```python
from build123d import *

# Parameters (mm, degrees)
BOSS_EXTRU_1_DEPTH      = 80
CONG_1_R                = 3
CONG_2_R                = 5
ENL_V_MAT_EXTRU_1_REACH = 119.218
ESQUISSE2_R             = 2.75
ENL_V_MAT_EXTRU_2_REACH = 116.084
ESQUISSE3_R             = 6.25
ENL_V_MAT_EXTRU_3_REACH = 125.629
ESQUISSE4_R             = 2.75
ENL_V_MAT_EXTRU_4_REACH = 122.661
ESQUISSE5_R             = 6.25
ENL_V_START             = -3.408092413
ENL_V_MAT_EXTRU_5_DEPTH = 3.408092413


# Read off the part's stored shape, not the designer's step: Enlèv. mat.-Extru.5
with BuildPart() as part:
    # Esquisse1 → Boss.-Extru.1 (new body)
    with BuildSketch(Plane.XY):
        Polygon((-33.585720943, 17.910660079), (-33.585720943, -57.089339921), (-28.585720943, -57.089339921), (41.414279057, 12.910660079), (41.414279057, 17.910660079), align=None)
        Polygon((-28.585720943, -52.269569409), (-28.585720943, 12.910660079), (36.594508545, 12.910660079), align=None, mode=Mode.SUBTRACT)
    extrude(amount=BOSS_EXTRU_1_DEPTH)

    # Congé1
    cong_1_edges = [part.edges().sort_by_distance(p)[0] for p in [
        (-28.585720943, -52.269569409, 40),
        (36.594508545, 12.910660079, 40),
    ]]
    fillet(cong_1_edges, radius=CONG_1_R)

    # Congé2
    cong_2_edges = [part.edges().sort_by_distance(p)[0] for p in [
        (-28.585720943, 12.910660079, 40),
    ]]
    fillet(cong_2_edges, radius=CONG_2_R)

    # Esquisse2 → Enlèv. mat.-Extru.1 (cut, up to next)
    with BuildSketch(Plane(origin=(0, 17.910660079, 0), x_dir=(1, 0, 0), z_dir=(0, 1, 0)), mode=Mode.PRIVATE) as enl_v_mat_extru_1_sk1:
        with Locations(Location((-13.585720943, -10, 0), (0, 0, 180))):
            Circle(ESQUISSE2_R)
    enl_v_mat_extru_1_tool1 = extrude(enl_v_mat_extru_1_sk1.sketch, amount=-ENL_V_MAT_EXTRU_1_REACH, mode=Mode.PRIVATE) & part.part
    # Esquisse2 → Enlèv. mat.-Extru.1 (cut, up to next)
    with BuildSketch(Plane(origin=(0, 17.910660079, 0), x_dir=(1, 0, 0), z_dir=(0, 1, 0)), mode=Mode.PRIVATE) as enl_v_mat_extru_1_sk2:
        with Locations(Location((31.414279057, -10, 0), (0, 0, 180))):
            Circle(ESQUISSE2_R)
    enl_v_mat_extru_1_tool2 = extrude(enl_v_mat_extru_1_sk2.sketch, amount=-ENL_V_MAT_EXTRU_1_REACH, mode=Mode.PRIVATE) & part.part
    # Esquisse2 → Enlèv. mat.-Extru.1 (cut, up to next)
    with BuildSketch(Plane(origin=(0, 17.910660079, 0), x_dir=(1, 0, 0), z_dir=(0, 1, 0)), mode=Mode.PRIVATE) as enl_v_mat_extru_1_sk3:
        with Locations(Location((31.414279057, -70, 0), (0, 0, 180))):
            Circle(ESQUISSE2_R)
    enl_v_mat_extru_1_tool3 = extrude(enl_v_mat_extru_1_sk3.sketch, amount=-ENL_V_MAT_EXTRU_1_REACH, mode=Mode.PRIVATE) & part.part
    # Esquisse2 → Enlèv. mat.-Extru.1 (cut, up to next)
    with BuildSketch(Plane(origin=(0, 17.910660079, 0), x_dir=(1, 0, 0), z_dir=(0, 1, 0)), mode=Mode.PRIVATE) as enl_v_mat_extru_1_sk4:
        with Locations(Location((-13.585720943, -70, 0), (0, 0, 180))):
            Circle(ESQUISSE2_R)
    enl_v_mat_extru_1_tool4 = extrude(enl_v_mat_extru_1_sk4.sketch, amount=-ENL_V_MAT_EXTRU_1_REACH, mode=Mode.PRIVATE) & part.part
    add(enl_v_mat_extru_1_tool1.solids().sort_by_distance((-13.585721, 17.91066, 10))[0], mode=Mode.SUBTRACT)
    add(enl_v_mat_extru_1_tool2.solids().sort_by_distance((31.414279, 17.91066, 10))[0], mode=Mode.SUBTRACT)
    add(enl_v_mat_extru_1_tool3.solids().sort_by_distance((31.414279, 17.91066, 70))[0], mode=Mode.SUBTRACT)
    add(enl_v_mat_extru_1_tool4.solids().sort_by_distance((-13.585721, 17.91066, 70))[0], mode=Mode.SUBTRACT)

    # Enlèv. mat.-Extru.2: up to this plane
    enl_v_mat_extru_2_end = Plane(origin=(-28.585720943, -57.089339921, 80), z_dir=(-0.7071067811865477, 0.7071067811865474, 0))
    # Esquisse3 → Enlèv. mat.-Extru.2 (cut, up to the surface)
    with BuildSketch(Plane.XZ.offset(-12.910660079), mode=Mode.PRIVATE) as enl_v_mat_extru_2_sk1:
        with Locations((-13.585720943, 10)):
            Circle(ESQUISSE3_R)
    enl_v_mat_extru_2_tool1 = split(extrude(enl_v_mat_extru_2_sk1.sketch, amount=ENL_V_MAT_EXTRU_2_REACH, mode=Mode.PRIVATE), bisect_by=enl_v_mat_extru_2_end, keep=Keep.BOTH, mode=Mode.PRIVATE)
    add(enl_v_mat_extru_2_tool1.solids().sort_by_distance((-13.585721, 12.91066, 10))[0], mode=Mode.SUBTRACT)
    # Esquisse3 → Enlèv. mat.-Extru.2 (cut, up to the surface)
    with BuildSketch(Plane.XZ.offset(-12.910660079), mode=Mode.PRIVATE) as enl_v_mat_extru_2_sk2:
        with Locations((-13.585720943, 70)):
            Circle(ESQUISSE3_R)
    enl_v_mat_extru_2_tool2 = split(extrude(enl_v_mat_extru_2_sk2.sketch, amount=ENL_V_MAT_EXTRU_2_REACH, mode=Mode.PRIVATE), bisect_by=enl_v_mat_extru_2_end, keep=Keep.BOTH, mode=Mode.PRIVATE)
    add(enl_v_mat_extru_2_tool2.solids().sort_by_distance((-13.585721, 12.91066, 70))[0], mode=Mode.SUBTRACT)
    # Esquisse3 → Enlèv. mat.-Extru.2 (cut, up to the surface)
    with BuildSketch(Plane.XZ.offset(-12.910660079), mode=Mode.PRIVATE) as enl_v_mat_extru_2_sk3:
        with Locations(Location((31.414279057, 10, 0), (0, 0, 109.267913115))):
            Circle(ESQUISSE3_R)
    enl_v_mat_extru_2_tool3 = split(extrude(enl_v_mat_extru_2_sk3.sketch, amount=ENL_V_MAT_EXTRU_2_REACH, mode=Mode.PRIVATE), bisect_by=enl_v_mat_extru_2_end, keep=Keep.BOTH, mode=Mode.PRIVATE)
    add(enl_v_mat_extru_2_tool3.solids().sort_by_distance((31.414279, 12.91066, 10))[0], mode=Mode.SUBTRACT)
    # Esquisse3 → Enlèv. mat.-Extru.2 (cut, up to the surface)
    with BuildSketch(Plane.XZ.offset(-12.910660079), mode=Mode.PRIVATE) as enl_v_mat_extru_2_sk4:
        with Locations(Location((31.414279057, 70, 0), (0, 0, 109.267913115))):
            Circle(ESQUISSE3_R)
    enl_v_mat_extru_2_tool4 = split(extrude(enl_v_mat_extru_2_sk4.sketch, amount=ENL_V_MAT_EXTRU_2_REACH, mode=Mode.PRIVATE), bisect_by=enl_v_mat_extru_2_end, keep=Keep.BOTH, mode=Mode.PRIVATE)
    add(enl_v_mat_extru_2_tool4.solids().sort_by_distance((31.414279, 12.91066, 70))[0], mode=Mode.SUBTRACT)

    # Esquisse4 → Enlèv. mat.-Extru.3 (cut, up to next)
    with BuildSketch(Plane.ZY.offset(33.585720943), mode=Mode.PRIVATE) as enl_v_mat_extru_3_sk1:
        with Locations(Location((10, -47.089339921, 0), (0, 0, 270))):
            Circle(ESQUISSE4_R)
    enl_v_mat_extru_3_tool1 = extrude(enl_v_mat_extru_3_sk1.sketch, amount=-ENL_V_MAT_EXTRU_3_REACH, mode=Mode.PRIVATE) & part.part
    # Esquisse4 → Enlèv. mat.-Extru.3 (cut, up to next)
    with BuildSketch(Plane.ZY.offset(33.585720943), mode=Mode.PRIVATE) as enl_v_mat_extru_3_sk2:
        with Locations(Location((10, -2.089339921, 0), (0, 0, 270))):
            Circle(ESQUISSE4_R)
    enl_v_mat_extru_3_tool2 = extrude(enl_v_mat_extru_3_sk2.sketch, amount=-ENL_V_MAT_EXTRU_3_REACH, mode=Mode.PRIVATE) & part.part
    # Esquisse4 → Enlèv. mat.-Extru.3 (cut, up to next)
    with BuildSketch(Plane.ZY.offset(33.585720943), mode=Mode.PRIVATE) as enl_v_mat_extru_3_sk3:
        with Locations(Location((70, -2.089339921, 0), (0, 0, 270))):
            Circle(ESQUISSE4_R)
    enl_v_mat_extru_3_tool3 = extrude(enl_v_mat_extru_3_sk3.sketch, amount=-ENL_V_MAT_EXTRU_3_REACH, mode=Mode.PRIVATE) & part.part
    # Esquisse4 → Enlèv. mat.-Extru.3 (cut, up to next)
    with BuildSketch(Plane.ZY.offset(33.585720943), mode=Mode.PRIVATE) as enl_v_mat_extru_3_sk4:
        with Locations(Location((70, -47.089339921, 0), (0, 0, 270))):
            Circle(ESQUISSE4_R)
    enl_v_mat_extru_3_tool4 = extrude(enl_v_mat_extru_3_sk4.sketch, amount=-ENL_V_MAT_EXTRU_3_REACH, mode=Mode.PRIVATE) & part.part
    add(enl_v_mat_extru_3_tool1.solids().sort_by_distance((-33.585721, -47.08934, 10))[0], mode=Mode.SUBTRACT)
    add(enl_v_mat_extru_3_tool2.solids().sort_by_distance((-33.585721, -2.08934, 10))[0], mode=Mode.SUBTRACT)
    add(enl_v_mat_extru_3_tool3.solids().sort_by_distance((-33.585721, -2.08934, 70))[0], mode=Mode.SUBTRACT)
    add(enl_v_mat_extru_3_tool4.solids().sort_by_distance((-33.585721, -47.08934, 70))[0], mode=Mode.SUBTRACT)

    # Esquisse5 → Enlèv. mat.-Extru.4 (cut, up to next)
    with BuildSketch(Plane(origin=(-28.585720943, 0, 0), x_dir=(0, 0, -1), z_dir=(1, 0, 0)), mode=Mode.PRIVATE) as enl_v_mat_extru_4_sk1:
        with Locations((-10, -2.089339921)):
            Circle(ESQUISSE5_R)
    enl_v_mat_extru_4_tool1 = extrude(enl_v_mat_extru_4_sk1.sketch, amount=ENL_V_MAT_EXTRU_4_REACH, mode=Mode.PRIVATE) & part.part
    # Esquisse5 → Enlèv. mat.-Extru.4 (cut, up to next)
    with BuildSketch(Plane(origin=(-28.585720943, 0, 0), x_dir=(0, 0, -1), z_dir=(1, 0, 0)), mode=Mode.PRIVATE) as enl_v_mat_extru_4_sk2:
        with Locations((-70, -2.089339921)):
            Circle(ESQUISSE5_R)
    enl_v_mat_extru_4_tool2 = extrude(enl_v_mat_extru_4_sk2.sketch, amount=ENL_V_MAT_EXTRU_4_REACH, mode=Mode.PRIVATE) & part.part
    # Esquisse5 → Enlèv. mat.-Extru.4 (cut, up to next)
    with BuildSketch(Plane(origin=(-28.585720943, 0, 0), x_dir=(0, 0, -1), z_dir=(1, 0, 0)), mode=Mode.PRIVATE) as enl_v_mat_extru_4_sk3:
        with Locations((-10, -47.089339921)):
            Circle(ESQUISSE5_R)
    enl_v_mat_extru_4_tool3 = extrude(enl_v_mat_extru_4_sk3.sketch, amount=ENL_V_MAT_EXTRU_4_REACH, mode=Mode.PRIVATE) & part.part
    # Esquisse5 → Enlèv. mat.-Extru.4 (cut, up to next)
    with BuildSketch(Plane(origin=(-28.585720943, 0, 0), x_dir=(0, 0, -1), z_dir=(1, 0, 0)), mode=Mode.PRIVATE) as enl_v_mat_extru_4_sk4:
        with Locations((-70, -47.089339921)):
            Circle(ESQUISSE5_R)
    enl_v_mat_extru_4_tool4 = extrude(enl_v_mat_extru_4_sk4.sketch, amount=ENL_V_MAT_EXTRU_4_REACH, mode=Mode.PRIVATE) & part.part
    add(enl_v_mat_extru_4_tool1.solids().sort_by_distance((-28.585721, -2.08934, 10))[0], mode=Mode.SUBTRACT)
    add(enl_v_mat_extru_4_tool2.solids().sort_by_distance((-28.585721, -2.08934, 70))[0], mode=Mode.SUBTRACT)
    add(enl_v_mat_extru_4_tool3.solids().sort_by_distance((-28.585721, -47.08934, 10))[0], mode=Mode.SUBTRACT)
    add(enl_v_mat_extru_4_tool4.solids().sort_by_distance((-28.585721, -47.08934, 70))[0], mode=Mode.SUBTRACT)

    # Enlèv. mat.-Extru.5 outline → Enlèv. mat.-Extru.5 (cut)
    with BuildSketch(Plane(origin=(14.251809489, -14.251809489, 0), x_dir=(0, 0, -1), z_dir=(0.7071067811865477, -0.7071067811865474, 0)).offset(ENL_V_START)):
        Polygon((-3.876275643, 15.432562462), (-3.75, 17.200329415), (-3.75, 24.271397227), (-3.876275643, 26.03916418), (-16.123724357, 26.03916418), (-16.25, 24.271397227), (-16.25, 17.200329415), (-16.123724357, 15.432562462), align=None)
        Polygon((-3.75, -46.439280892), (-3.75, -39.36821308), (-3.876275643, -37.600446127), (-16.123724357, -37.600446127), (-16.25, -39.36821308), (-16.25, -46.439280892), (-16.123724357, -48.207047845), (-3.876275643, -48.207047845), align=None)
        Polygon((-76.123724357, -37.600446127), (-76.25, -39.36821308), (-76.25, -46.439280892), (-76.123724357, -48.207047845), (-63.876275643, -48.207047845), (-63.75, -46.439280892), (-63.75, -39.36821308), (-63.876275643, -37.600446127), align=None)
        Polygon((-63.876275643, 15.432562462), (-63.75, 17.200329415), (-63.75, 24.271397227), (-63.876275643, 26.03916418), (-76.123724357, 26.03916418), (-76.25, 24.271397227), (-76.25, 17.200329415), (-76.123724357, 15.432562462), align=None)
    extrude(amount=ENL_V_MAT_EXTRU_5_DEPTH, mode=Mode.SUBTRACT)


solid = part.part
```
Geometry check sheet. Reference: the model listing, model coordinates, mm. A direction names the side the tool comes from. Give positions to 0.01 mm unless a question says otherwise; leave off trailing zeros. Write each loop counter-clockwise with the first axis right and the second up, starting at its lowest first coordinate (ties: lowest second). Pieces come first, ordered by that corner, then holes. Notation, with made-up numbers: (40.5, 34) -> (79.5, 34) arc R18 cw to (79.5, 39) -> close; hole circle Ø11 at (18.5, -13.75). An arc over 180 degrees is marked (long way). One line per question, with ' | ' between items.
Item 1: Sectioned sample at B-B, the plane y = -16.5. Record the boundary of the cut face in (x, z), plus the area to 3 significant figures.
Determined:
outline: (-33.59, 0) -> (-28.59, 0) -> (-28.59, 80) -> (-33.59, 80) -> close; (7.18, 0) -> (12, 0) -> (12, 80) -> (7.18, 80) -> close | area: 786 mm^2
Item 2: Depth check by flat-ended pin: pin 1 (1.5 mm diameter, centred on y = -11.5, z = 12, fed in from +X); pin 2 (7 mm diameter, centred on y = -47.09, z = 70, fed in from +X). Enter the tip coordinate at first touch or a pass-through.
Determined:
pin 1: x = 17.75 | pin 2: x = -28.59
Item 3: Sectioned sample at A-A, the plane z = 51.5. Record the boundary of the cut face in (x, y), plus the area to 3 significant figures.
Determined:
outline: (-33.59, -57.09) -> (-28.59, -57.09) -> (41.41, 12.91) -> (41.41, 17.91) -> (-33.59, 17.91) -> close; hole (-28.59, -45.03) arc R3 ccw to (-23.46, -47.15) -> (31.47, 7.79) arc R3 ccw to (29.35, 12.91) -> (-23.59, 12.91) arc R5 ccw to (-28.59, 7.91) -> close | area: 1,080 mm^2
Item 4: Access from +Z, -Z, +X, -X, +Y, -Y to the whole of each face (thin tool, end or side, straight path). Record for faces 1 (the flat face through (29.996, 5.007, 76.216)), 2 (the flat face through (24.335, -0.654, 16.217)), 3 (the cylindrical face through (32.142, 11.013, 2.079)).
Determined:
face 1: -Y | face 2: +X | face 3: +Z, -Z
Item 5: Sectioned sample at C-C, the plane z = 70. State how many separate pieces and enclosed holes the cut face has, plus the area to 3 significant figures.
Determined:
separate pieces: 6 | enclosed holes: 0 | area: 755 mm^2
Item 6: Sectioned sample at D-D, the plane x = 6.5. Record the boundary of the cut face in (y, z), plus the area to 3 significant figures.
Determined:
outline: (-22, 0) -> (-17.18, 0) -> (-17.18, 80) -> (-22, 80) -> close; (12.91, 0) -> (17.91, 0) -> (17.91, 80) -> (12.91, 80) -> close | area: 786 mm^2
Item 7: Scan lines: line 1 along Z through (x, y) = (-25, -51); line 2 along X through (y, z) = (-30.5, 48); line 3 along Y through (x, z) = (19, 34). Record each from-to range of solid material in increasing order.
Determined:
line 1: 0 to 5.12, 14.88 to 65.12, 74.88 to 80 | line 2: -33.59 to -28.59, -6.82 to -2 | line 3: -9.5 to -4.68, 12.91 to 17.91
Item 8: Draft check along X on faces 4 (the flat face through (41.414, 15, 39)), 5 (the cylindrical face through (-13.228, 15.446, 72.727)), 6 (the cylindrical face through (-31.1, -45.1, 71.9)). Enter one of: released by +X, released by -X, zero draft, split by the parting line, or undercut.
Determined:
face 4: released by +X | face 5: undercut | face 6: zero draft
